The model under review builds one solid part; all positions refer to its coordinate system, in mm. Face numbers are marked on the shaded views. Coordinates: 2 decimals unless noted, no trailing zeros. Write each loop counter-clockwise with the first axis right and the second up, starting at its lowest first coordinate (ties: lowest second). Pieces come first, ordered by that corner, then holes. Notation, with made-up numbers: (-4, 27.25) -> (53, 27.25) arc R17 ccw to (53, 54.25) -> close; hole circle Ø6 at (-11.5, 50.25). An arc over 180 degrees is marked (long way). Write each question's results on one line, items separated by ' | '.
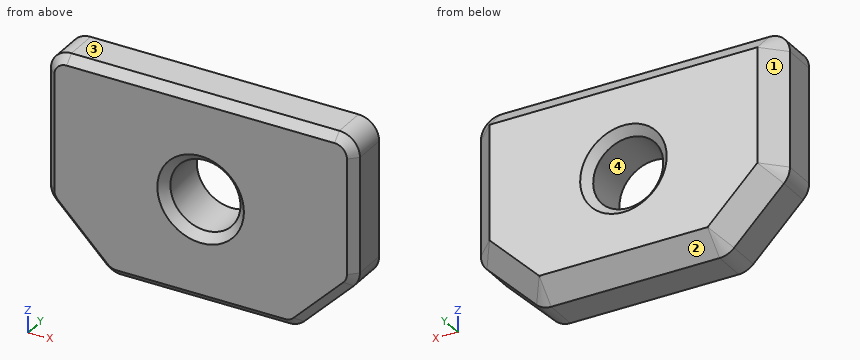
Autodesk Fusion 360 part; units mm, degrees
sketch "Sketch1" plane through (0, 0, 0) normal (0, 1, 0) x (1, 0, 0) in component "[a]_Railstops_x6"
  line L0 (7.5, 5) -> (-7.5, 5)
  line L1 (-7.5, 5) -> (-7.5, -5)
  line L2 (-7.5, -5) -> (7.5, -5)
  line L3 (7.5, -5) -> (7.5, 5)
  line L4 (7.5, 5) -> (-7.5, -5) construction
  line L5 (-7.5, 5) -> (7.5, -5) construction
  dimension "d1" = 15
  dimension "d2" = 10
extrude "Extrude1" add sketch "Sketch1" along normal mid plane 3 in component "[a]_Railstops_x6"
chamfer "Chamfer1" distance 3 angle 45 2 edges at (-7.5, 0, -5) (7.5, 0, -5) measured on face at (-2.5, 0.5, -5) measured on face at (7.5, -0.5, 1.6667) in component "[a]_Railstops_x6"
fillet "Fillet1" radius 1 6 edges at (7.5, 0, 5) (-7.5, 0, 5) (-7.5, 0, -2) (-4.5, 0, -5) (4.5, 0, -5) (7.5, 0, -2) in component "[a]_Railstops_x6"
chamfer "Chamfer2" distance 0.4 angle 45 1 faces at (-1.3619, -1.5, 1.6667) in component "[a]_Railstops_x6"
chamfer "Chamfer2" distance 1 angle 45 1 faces at (-1.3619, 1.5, 1.6667) in component "[a]_Railstops_x6"
sketch "Sketch2" plane through (0, -1.5, 0) normal (0, -1, 0) x (1, 0, 0) in component "[a]_Railstops_x6"
  arc A0 (6.9243, -2.0101) -> (7.1, -1.5858) centre (6.5, -1.5858) ccw
  line L0 (7.1, -1.5858) -> (7.1, 4)
  arc A1 (7.1, 4) -> (6.5, 4.6) centre (6.5, 4) ccw
  line L1 (6.5, 4.6) -> (-6.5, 4.6)
  arc A2 (-6.5, 4.6) -> (-7.1, 4) centre (-6.5, 4) ccw
  line L2 (-7.1, 4) -> (-7.1, -1.5858)
  arc A3 (-7.1, -1.5858) -> (-6.9243, -2.0101) centre (-6.5, -1.5858) ccw
  line L3 (-6.9243, -2.0101) -> (-4.5101, -4.4243)
  arc A4 (-4.5101, -4.4243) -> (-4.0858, -4.6) centre (-4.0858, -4) ccw
  line L4 (-4.0858, -4.6) -> (4.0858, -4.6)
  arc A5 (4.0858, -4.6) -> (4.5101, -4.4243) centre (4.0858, -4) ccw
  line L5 (4.5101, -4.4243) -> (6.9243, -2.0101)
  line L6 (0, 0) -> (0, 7) construction
  point P0 (0, 0.5)
  dimension "d16" = 0.5
hole "Hole1" at (0, -1.5, 0) direction (0, 1, 0) diameter 3.4 end through all in component "[a]_Railstops_x6"
chamfer "Chamfer3" distance 0.4 angle 45 2 edges at (0.6147, -1.5, 1.585) (-0.6147, 1.5, 1.585) measured on face at (-5.2858, -1.5, 0.9308) measured on face at (4.8858, 1.5, 0.9308) in component "[a]_Railstops_x6"
component "[a]_Railstops_x6" placed x (1, 0, 0) y (0, 1, 0) z (0, 0, 1) at (0, 0, 0)
Q1. For line 1 (Z direction, x = 0, y = -0.3); line 2 (X direction, y = 0.25, z = 0); line 3 (X direction, y = 0.6, z = 0), list the stretches that pass through material, from the lowest coordinate up. Write a range as from..to.
Solution:
line 1: -5..-1.7, 1.7..5 | line 2: -7.5..-1.7, 1.7..7.5 | line 3: -7.4..-1.7, 1.7..7.4
Q2. Add section A-A (z = 0). Write out the cut boundary in (x, y), plus the area to 3 significant figures.
Solution:
outline: (-7.5, -1.1) -> (-7.1, -1.5) -> (-2.1, -1.5) -> (-1.7, -1.1) -> (-1.7, 1.1) -> (-2.1, 1.5) -> (-6.5, 1.5) -> (-7.5, 0.5) -> close; (1.7, -1.1) -> (2.1, -1.5) -> (7.1, -1.5) -> (7.5, -1.1) -> (7.5, 0.5) -> (6.5, 1.5) -> (2.1, 1.5) -> (1.7, 1.1) -> close | area: 33.3 mm²
Q3. Add section D-D (z = 3.5). Write out the cut boundary in (x, y).
Solution:
outline: (-7.5, -1.1) -> (-7.1, -1.5) -> (7.1, -1.5) -> (7.5, -1.1) -> (7.5, 0.5) -> (6.5, 1.5) -> (-6.5, 1.5) -> (-7.5, 0.5) -> close
Q4. Add section B-B (y = 0). Write out the cut boundary in (x, z).
Solution:
outline: (-7.5, -1.59) arc R1 ccw to (-7.21, -2.29) -> (-4.79, -4.71) arc R1 ccw to (-4.09, -5) -> (4.09, -5) arc R1 ccw to (4.79, -4.71) -> (7.21, -2.29) arc R1 ccw to (7.5, -1.59) -> (7.5, 4) arc R1 ccw to (6.5, 5) -> (-6.5, 5) arc R1 ccw to (-7.5, 4) -> close; hole circle Ø3.4 at (0, 0)
Q5. Draft analysis for pull direction Z (two halves, no side actions). For the marked faces 1, 2, 3 and 4, state which applies: pulls with the +Z half, pulls with the -Z half, needs draft (parallel to the pull), parting line crosses it, or undercut.
Solution:
face 1: needs draft | face 2: pulls with the -Z half | face 3: pulls with the +Z half | face 4: undercut
Q6. Add section C-C (x = 0). Write out the cut boundary in (y, z).
Solution:
outline: (-1.5, -4.6) -> (-1.1, -5) -> (0.5, -5) -> (1.5, -4) -> (1.5, -2.1) -> (1.1, -1.7) -> (-1.1, -1.7) -> (-1.5, -2.1) -> close; (-1.5, 2.1) -> (-1.1, 1.7) -> (1.1, 1.7) -> (1.5, 2.1) -> (1.5, 4) -> (0.5, 5) -> (-1.1, 5) -> (-1.5, 4.6) -> close
